Source: CAD feature listing. Evaluate the final solid. Frame: model axes, mm. A direction names the side the tool comes from. Give positions to 0.01 mm unless a question says otherwise; leave off trailing zeros. Write each loop counter-clockwise with the first axis right and the second up, starting at its lowest first coordinate (ties: lowest second). Pieces come first, ordered by that corner, then holes. Notation, with made-up numbers: M 73,22 L 117,22 A24 ccw 117,59 Z; hole C 62.5,-5 d9. An arc over 180 degrees is marked long. Answer as a JSON object with one key per item and string values. Group by question number.
```python
from build123d import *

# Parameters (mm, degrees)
F0_W     = 31.75
F0_H     = 50.8
F1_DEPTH = 25.4
F4_DEPTH = 31.751
F2_W     = 19.05
F2_H     = 19.05
F5_DEPTH = 50.546


with BuildPart() as f1:
    # F0 (on Front) → F1 (new body)
    with BuildSketch(Plane.XZ):
        with Locations((-37.953461, 60.855525)):
            Rectangle(F0_W, F0_H)
    extrude(amount=F1_DEPTH)

    # F3 (on face) → F4 (cut, through all)
    with BuildSketch(Plane.YZ.offset(-22.078461)):
        Polygon((-25.4, 54.505525), (0, 86.255525), (-25.4, 86.255525), align=None)
    extrude(amount=-F4_DEPTH, mode=Mode.SUBTRACT)

    # F2 (on face) → F5 (join)
    with BuildSketch(Plane.XY.offset(86.255525)):
        with Locations((-44.303461, -9.525)):
            Rectangle(F2_W, F2_H)
    extrude(amount=-F5_DEPTH)


solid = f1.part
```
(1) Section C-C, the plane y = -17. Return loops of the section in (x, z), plus the area to 3 significant figures.
(2) Section A-A, the plane x = -23.5. Return loops of the section in (y, z), plus the area to 3 significant figures.
(3) Section D-D, the plane y = -23. Return loops of the section in (x, z).
(4) Contact query for flat-ended pins moving along their axis: pin 1 Ø12 at (x, z) = (-46, 79) entering from +Y; pin 2 Ø9.5 at (x, z) = (-45.5, 70) entering from -Y. Output: stop coordinate, or through.
(5) Access query for faces 1 (the flat face through (-44, -9, 86.256)), 2 (the flat face through (-34.778, -12, 77)), 3 (the flat face through (-44, -19.05, 75)). Directions: +Z, -Z, +X, -X, +Y, -Y. A direction counts if a zero-diameter tool reaches every point of the face in a straight line with its end or side. Return the directions, or none.
(6) Ray query, L1, parallel to Y at x = -43.5, z = 78; L2, parallel to X at y = -8.75, z = 76; L3, parallel to Z at x = -30.5, y = -14.5. Return the intervals inside material, ascending. Write a range as [from, to].
(7) Section B-B, the plane z = 65.5. Return loops of the section in (x, y), plus the area to 3 significant figures.
Reported:
{
 "1": {"outline": "M -53.83,35.46 L -22.08,35.46 L -22.08,65.01 L -34.78,65.01 L -34.78,86.26 L -53.83,86.26 Z", "area": "1,340 mm2"},
 "2": {"outline": "M -25.4,35.46 L 0,35.46 L 0,86.26 L -25.4,54.51 Z", "area": "887 mm2"},
 "3": {"outline": "M -53.83,35.46 L -22.08,35.46 L -22.08,57.51 L -53.83,57.51 Z"},
 "4": {"pin 1": "stops at y = 0", "pin 2": "stops at y = -19.05"},
 "5": {"face 1": "+Z, +X, -X, +Y, -Y", "face 2": "+Z, +X, -Y", "face 3": "+Z, +X, -X, -Y"},
 "6": {"L1": "y = [-19.05, 0]", "L2": "x = [-53.83, -34.78]", "L3": "z = [35.46, 68.13]"},
 "7": {"outline": "M -53.83,-19.05 L -34.78,-19.05 L -34.78,-16.6 L -22.08,-16.6 L -22.08,0 L -53.83,0 Z", "area": "574 mm2"}
}
